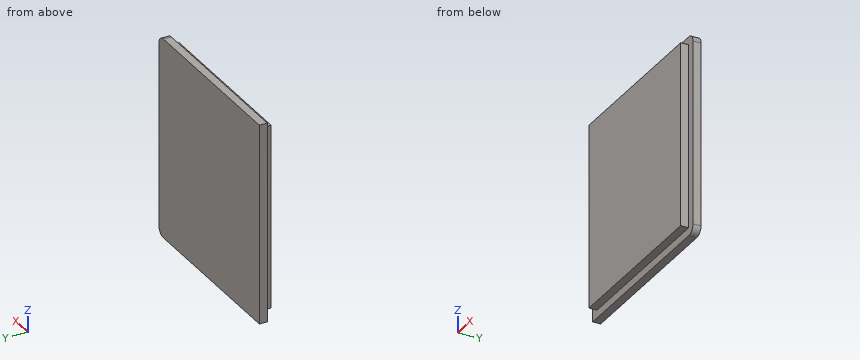
```python
from build123d import *

# Parameters (mm, degrees)
SKETCH1_W           = 70
SKETCH1_H           = 75
BOSS_EXTRUDE1_DEPTH = 3
SKETCH2_W           = 64
SKETCH2_H           = 69
BOSS_EXTRUDE2_DEPTH = 3
FILLET1_R           = 3


with BuildPart() as part:
    # Sketch1 → Boss-Extrude1 (new body)
    with BuildSketch(Plane(origin=(0, 0, 0), x_dir=(1, 0, 0), z_dir=(0, 1, 0))):
        Rectangle(SKETCH1_W, SKETCH1_H)
    extrude(amount=BOSS_EXTRUDE1_DEPTH)

    # Sketch2 → Boss-Extrude2 (add)
    with BuildSketch(Plane.XZ):
        Rectangle(SKETCH2_W, SKETCH2_H)
    extrude(amount=BOSS_EXTRUDE2_DEPTH)

    # Fillet1
    fillet1_edges = [part.edges().sort_by_distance(p)[0] for p in [
        (35, 1.5, 37.5),
        (35, 1.5, -37.5),
    ]]
    fillet(fillet1_edges, radius=FILLET1_R)


solid = part.part
```
Part model, mm, in its own coordinate system. Give positions to 0.01 mm unless a question says otherwise; leave off trailing zeros. Write each loop counter-clockwise with the first axis right and the second up, starting at its lowest first coordinate (ties: lowest second). Pieces come first, ordered by that corner, then holes. Notation, with made-up numbers: (89, -35) -> (144, -35) arc R31 ccw to (144, -11) -> close; hole circle Ø10 at (65.5, 14). An arc over 180 degrees is marked (long way). Put each result on its own line as item: value. Start each with the question number.
Item 1: Cut at B-B (x = -2.5). List the corners of the cut face in (y, z).
Item 2: Pin check, flat tips, straight feed: pin 1 Ø1 at (y, z) = (-2, -1) entering from +X; pin 2 Ø2.5 at (x, y) = (-16, -1.5) entering from -Z; pin 3 Ø0.9 at (y, z) = (-1.5, -6) entering from -X. Stop position of each tip, or through.
Item 3: Wall check: L1, parallel to Z at x = 10.5, y = -0.15; L2, parallel to X at y = -1.5, z = 0. Give the ranges that are in metal, low to high. Write a range as [from, to].
Item 4: Cut at A-A (z = 8.5). List the corners of the cut face in (x, y), then the cut area to 3 significant figures.
Item 5: Cut at C-C (y = -1.15). List the corners of the cut face in (x, z).
Answer list:
1. outline: (-3, -34.5) -> (0, -34.5) -> (0, -37.5) -> (3, -37.5) -> (3, 37.5) -> (0, 37.5) -> (0, 34.5) -> (-3, 34.5) -> close
2. pin 1: stops at x = 32
2. pin 2: stops at z = -34.5
2. pin 3: stops at x = -32
3. L1: z = [-34.5, 34.5]
3. L2: x = [-32, 32]
4. outline: (-35, 0) -> (-32, 0) -> (-32, -3) -> (32, -3) -> (32, 0) -> (35, 0) -> (35, 3) -> (-35, 3) -> close
4. area: 402 mm2
5. outline: (-32, -34.5) -> (32, -34.5) -> (32, 34.5) -> (-32, 34.5) -> close
